Geometry: final body of the model. Coordinates: model frame, mm. A direction names the side the tool comes from. Give positions to 0.01 mm unless a question says otherwise; leave off trailing zeros. Write each loop counter-clockwise with the first axis right and the second up, starting at its lowest first coordinate (ties: lowest second). Pieces come first, ordered by that corner, then holes.
Q1. Cut plane A-A on y = -8.5. Return the cut outline in (x, z), plus the area to 3 significant figures.
Q2. Reachability of faces 1 (the face through (0, -2, 27.75)), 2 (the face through (14, -0.5, 22)), 3 (the face through (8.85, -9, 27)), 4 (the face through (-12.75, 0, 24)), 5 (the face through (14.715, -9.699, 26.887)) from +Z, -Z, +X, -X, +Y, -Y: full face, straight path, thin tool, end or side. Return the list, or none.
Q3. Cut plane B-B on x = 7.25. Return the cut outline in (y, z), plus the area to 3 significant figures.
Q4. Line query: L1, parallel to Y at x = -4, z = 27; L2, parallel to X at y = -8.75, z = 26.25; L3, parallel to Y at x = -0.25, z = 22.25. Output: solid intervals per line, ascending.
Q5. Cut plane C-C on z = 22. Return the cut outline in (x, y).
Q6. Pin query (flat end, axial travel): pin 1 (1 mm diameter, centred on x = 9.5, y = -1.5, fed in from -Z); pin 2 (3 mm diameter, centred on x = -11.5, z = 24, fed in from -Y); pin 3 (3 mm diameter, centred on x = 9, z = 24, fed in from -Y). Return the tip coordinate at first contact, or that it passes through.
Q7. Cut plane D-D on z = 27. Return the cut outline in (x, y), plus the area to 3 significant figures.
Q8. Draft query along X for faces 6 (the face through (0, -10, 27)), 7 (the face through (15, 1, 24)), 8 (the face through (-7.3, -5.9, 26.9)). Return one class per face: pulls with the +X half, pulls with the -X half, needs draft (parallel to the pull), parting line crosses it, or undercut.
```python
from build123d import *

# Parameters (mm, degrees)
BOSS_EXTRUDE1_DEPTH      = 27.75
BOSS_EXTRUDE1_DEPTH_BACK = 27.75
SKETCH1_W                = 30
SKETCH1_H                = 15
SKETCH3_W                = 4
SKETCH3_H                = 18.5
CUT_EXTRUDE2_DEPTH       = 43.072110715
CUT_EXTRUDE5_DEPTH       = 3
CUT_EXTRUDE6_START       = -3
CUT_EXTRUDE6_DEPTH       = 3
FILLET1_R                = 1
SKETCH7_W                = 52
SKETCH7_H                = 19
CUT_EXTRUDE8_DEPTH       = 43.072110715
SKETCH8_W                = 25.5
SKETCH8_H                = 1.2
SKETCH8_H_2              = 1.187456806
CUT_EXTRUDE9_DEPTH       = 21.495426319


with BuildPart() as part:
    # Sketch1 → Boss-Extrude1 (new, two sides: drawn at the far end of the back side and taken through both)
    with BuildSketch(Plane.XY.offset(-BOSS_EXTRUDE1_DEPTH_BACK)):
        with Locations((0, -2.5)):
            Rectangle(SKETCH1_W, SKETCH1_H)
    extrude(amount=BOSS_EXTRUDE1_DEPTH + BOSS_EXTRUDE1_DEPTH_BACK)

    # Sketch3 → Cut-Extrude2 (cut, through all)
    with BuildSketch(Plane(origin=(15, 0, 0), x_dir=(0, 0, -1), z_dir=(1, 0, 0))):
        with Locations((24, -10)):
            Rectangle(SKETCH3_W, SKETCH3_H)
        with Locations((-24, -10)):
            Rectangle(SKETCH3_W, SKETCH3_H)
    extrude(amount=-CUT_EXTRUDE2_DEPTH, mode=Mode.SUBTRACT)

    # Sketch2 → Cut-Extrude5 (cut)
    with BuildSketch(Plane.XY.offset(27.75)):
        with BuildLine():
            Line((-8.85, -12.5), (-8.85, -7.5))
            ThreePointArc((-8.85, -7.5), (-7.25, -5.9), (-5.65, -7.5))
            Line((-5.65, -7.5), (-5.65, -12.5))
            ThreePointArc((-5.65, -12.5), (-7.25, -14.1), (-8.85, -12.5))
        make_face()
        with BuildLine():
            Line((5.65, -12.5), (5.65, -7.5))
            ThreePointArc((5.65, -7.5), (7.25, -5.9), (8.85, -7.5))
            Line((8.85, -7.5), (8.85, -12.5))
            ThreePointArc((8.85, -12.5), (7.25, -14.1), (5.65, -12.5))
        make_face()
    extrude(amount=-CUT_EXTRUDE5_DEPTH, mode=Mode.SUBTRACT)

    # Sketch5 → Cut-Extrude6 (cut)
    with BuildSketch(Plane(origin=(0, 0, -27.75), x_dir=(-1, 0, 0), z_dir=(0, 0, -1)).offset(CUT_EXTRUDE6_START)):
        with BuildLine():
            Line((-8.85, -12.5), (-8.85, -7.5))
            ThreePointArc((-8.85, -7.5), (-7.25, -5.9), (-5.65, -7.5))
            Line((-5.65, -7.5), (-5.65, -12.5))
            ThreePointArc((-5.65, -12.5), (-7.25, -14.1), (-8.85, -12.5))
        make_face()
        with BuildLine():
            Line((5.65, -12.5), (5.65, -7.5))
            ThreePointArc((5.65, -7.5), (7.25, -5.9), (8.85, -7.5))
            Line((8.85, -7.5), (8.85, -12.5))
            ThreePointArc((8.85, -12.5), (7.25, -14.1), (5.65, -12.5))
        make_face()
    extrude(amount=CUT_EXTRUDE6_DEPTH, mode=Mode.SUBTRACT)

    # Fillet1
    fillet1_edges = [part.edges().sort_by_distance(p)[0] for p in [
        (15, -10, 26.875),
    ]]
    fillet(fillet1_edges, radius=FILLET1_R)

    # Sketch7 → Cut-Extrude8 (cut, through all)
    with BuildSketch(Plane(origin=(15, 0, 0), x_dir=(0, 0, -1), z_dir=(1, 0, 0))):
        with Locations((0, -10)):
            Rectangle(SKETCH7_W, SKETCH7_H)
    extrude(amount=-CUT_EXTRUDE8_DEPTH, mode=Mode.SUBTRACT)

    # SurfaceCut1
    split(bisect_by=Plane.XY.offset(18), keep=Keep.TOP)

    # Sketch8 → Cut-Extrude9 (cut, through all)
    with BuildSketch(Plane.XY.offset(27.75)):
        with Locations((0, -0.4)):
            Rectangle(SKETCH8_W, SKETCH8_H)
        with Locations((0, 3.5)):
            Rectangle(SKETCH8_W, SKETCH8_H_2)
    extrude(amount=-CUT_EXTRUDE9_DEPTH, mode=Mode.SUBTRACT)


solid = part.part
```
Data:
1. outline: (-15, 26) - (-8.85, 26) - (-8.85, 27.75) - (-15, 27.75) - close; (-5.65, 26) - (5.65, 26) - (5.65, 27.75) - (-5.65, 27.75) - close; (8.85, 26) - (15, 26) - (15, 27.75) - (8.85, 27.75) - close
1. area: 41.3 mm2
2. face 1: +Z, +X, -X, +Y, -Y
2. face 2: -Z, +X, -X, -Y
2. face 3: +Z, -Z, -Y
2. face 4: +Z, -Z
2. face 5: +Z, -Z, +X, -Y
3. outline: (-5.9, 26) - (-1, 26) - (-1, 27.75) - (-5.9, 27.75) - close; (0.2, 18) - (2.91, 18) - (2.91, 27.75) - (0.2, 27.75) - close; (4.09, 18) - (5, 18) - (5, 27.75) - (4.09, 27.75) - close
3. area: 43.8 mm2
4. L1: y = -10 to -1, 0.2 to 2.91, 4.09 to 5
4. L2: x = -15 to -8.85, -5.65 to 5.65, 8.85 to 15
4. L3: y = 0.2 to 2.91, 4.09 to 5
5. outline: (-15, -0.5) - (-12.75, -0.5) - (-12.75, 0.2) - (12.75, 0.2) - (12.75, -0.5) - (15, -0.5) - (15, 5) - (-15, 5) - close; hole (-12.75, 2.91) - (12.75, 2.91) - (12.75, 4.09) - (-12.75, 4.09) - close
6. pin 1: stops at z = 26
6. pin 2: stops at y = -0.5
6. pin 3: stops at y = 0.2
7. outline: (-15, -10) - (-8.85, -10) - (-8.85, -7.5) arc R1.6 cw to (-5.65, -7.5) - (-5.65, -10) - (5.65, -10) - (5.65, -7.5) arc R1.6 cw to (8.85, -7.5) - (8.85, -10) - (14, -10) arc R1 ccw to (15, -9) - (15, 5) - (-15, 5) - close; hole (-12.75, -1) - (12.75, -1) - (12.75, 0.2) - (-12.75, 0.2) - close; hole (-12.75, 2.91) - (12.75, 2.91) - (12.75, 4.09) - (-12.75, 4.09) - close
7. area: 365 mm2
8. face 6: needs draft
8. face 7: pulls with the +X half
8. face 8: undercut
